Here's the drawing with two shaded views (mm, measured from the low corner). I have some questions. A direction names the side the tool comes from. Give positions to 0.01 mm unless a question says otherwise; leave off trailing zeros. Loops run counter-clockwise (first coordinate to the right, second up) from the corner with the lowest first, then second, coordinate; pieces in that order, holes last. Notation, with made-up numbers: M -1,61.25 L 49,61.25 A13 cw 49,75.25 Z; hole C 39,0 d6. An arc over 180 degrees is marked long. Use CSV: the item, a comma, the result in double quotes.
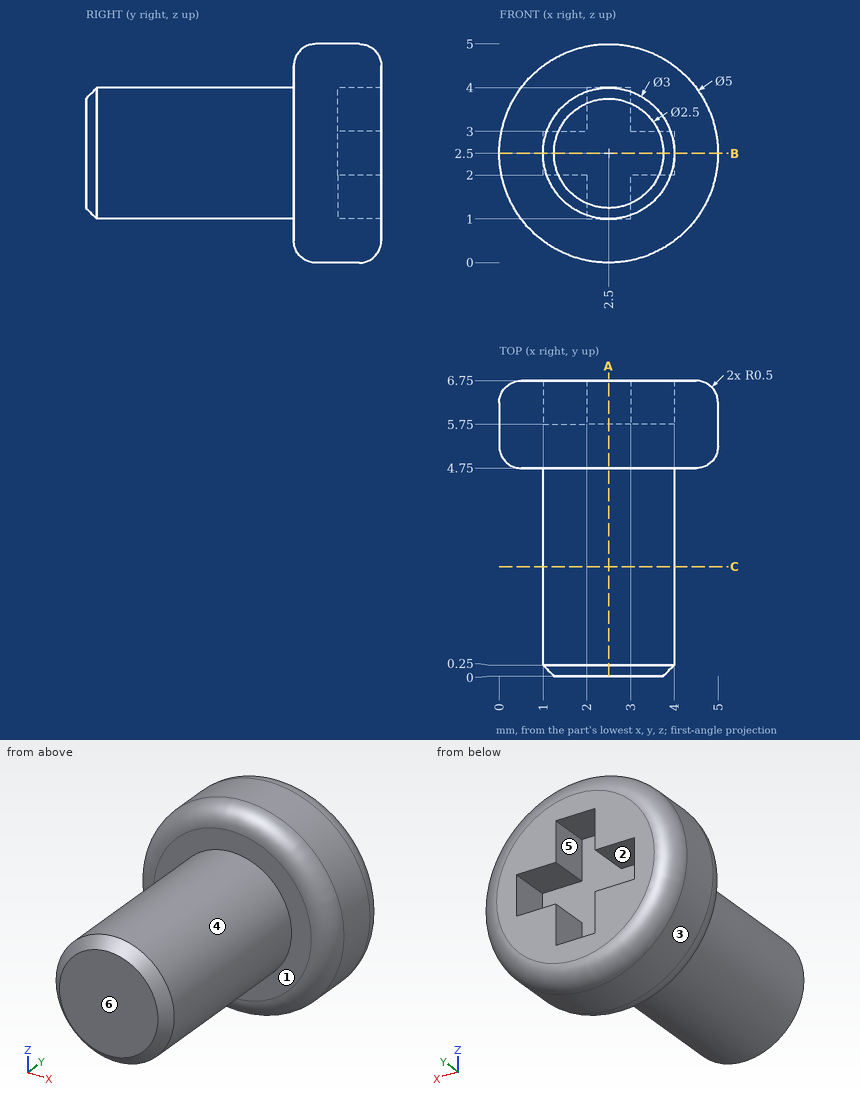
1. I'm going to push flat-ended pins straight in: pin 1 Ø0.8 at (y, z) = (6.5, 1.5) entering from -X; pin 2 Ø1 at (x, y) = (1.5, 3) entering from -Z; pin 3 Ø0.8 at (x, y) = (3.5, 6) entering from -Z; pin 4 Ø1.1 at (y, z) = (6.5, 2.5) entering from +X. Where does each tip first touch, or does it pass through?
Outcome:
pin 1,"x = 0.09"
pin 2,"z = 1.09"
pin 3,"z = 0.07"
pin 4,"x = 5"
2. I want a section at B-B, the plane z = 2.5. List the corners of the cut face in (x, y) for me.
Outcome:
outline,"M 0,5.25 A0.5 ccw 0.5,4.75 L 1,4.75 L 1,0.25 L 1.25,0 L 3.75,0 L 4,0.25 L 4,4.75 L 4.5,4.75 A0.5 ccw 5,5.25 L 5,6.25 A0.5 ccw 4.5,6.75 L 4,6.75 L 4,5.75 L 1,5.75 L 1,6.75 L 0.5,6.75 A0.5 ccw 0,6.25 Z"
3. Please list where these lines run through material, in increasing order: line 1 (Y direction, x = 3.4, z = 4); line 2 (Z direction, x = 0.5, y = 6); line 3 (Z direction, x = 2.2, y = 6).
Outcome:
line 1,"4.75 to 6.75"
line 2,"1 to 4"
line 3,"0.02 to 1, 4 to 4.98"
4. Which directions (+Z, -Z, +X, -X, +Y, -Y) give clear straight access to the entire face, cutting with the end or side of a thin tool? Please do the marked faces 4, 5 and 6.
Outcome:
face 4,"-Y"
face 5,"+Y"
face 6,"+Z, -Z, +X, -X, -Y"
5. I want a section at A-A, the plane x = 2.5. List the corners of the cut face in (y, z) for me.
Outcome:
outline,"M 0,1.25 L 0.25,1 L 4.75,1 L 4.75,0.5 A0.5 ccw 5.25,0 L 6.25,0 A0.5 ccw 6.75,0.5 L 6.75,1 L 5.75,1 L 5.75,4 L 6.75,4 L 6.75,4.5 A0.5 ccw 6.25,5 L 5.25,5 A0.5 ccw 4.75,4.5 L 4.75,4 L 0.25,4 L 0,3.75 Z"
6. If we mould it in two halves opening along X, with no side actions, what happens to the marked faces 1, 2 and 3? For each: +X half, -X half, draft (parallel to the pull), parting line (faces both ways), or undercut.
Outcome:
face 1,"draft"
face 2,"undercut"
face 3,"parting line"
7. I want a section at C-C, the plane y = 2.5. List the corners of the cut face in (x, z) for me, then the cut area to 3 significant figures.
Outcome:
outline,"C 2.5,2.5 d3"
area,"7.07 mm2"
